Design review of the part built by this model. Coordinates are the model's own, in mm. A direction names the side the tool comes from. Give positions to 0.01 mm unless a question says otherwise; leave off trailing zeros. Loops run counter-clockwise (first coordinate to the right, second up) from the corner with the lowest first, then second, coordinate; pieces in that order, holes last. Notation, with made-up numbers: (-12, 63) -> (-1, 63) arc R18 ccw to (-1, 94) -> close; hole circle Ø9 at (78.5, 58). An arc over 180 degrees is marked (long way). Use a Markdown table: item, result. Add a question column.
1. For faces 1 (the flat face through (-256.279, 10.628, -40.025)), 2 (the cylindrical face through (-281.7, 4.2, -4)), list the 3-axis set-ups (+Z, -Z, +X, -X, +Y, -Y) from which the entire face can be reached by the end or side of a thin tool; tool diameter is ignored.
2. Add section A-A (x = -155). State the section outline as (y, z) points, and give its area (3 significant figures).
3. For pin 1 Ø0.9 at (x, y) = (-274.5, 24) entering from +Z; pin 2 Ø10 at (x, y) = (-470.5, 8) entering from +Z; pin 3 Ø12 at (x, z) = (-63, -6) entering from -Y, all flat-tipped, find the tip position at first contact; note any pin that passes through.
4. To check wall thickness, follow line 1 (Y direction, x = -477.5, z = -13); line 2 (Y direction, x = -232, z = -1.5); line 3 (X direction, y = 12.5, z = -14.5). State the ranges of each line that lie inside material, in increasing order.
```python
from build123d import *

# Parameters (mm, degrees)
F1_DEPTH      = 41
F1_DEPTH_BACK = 824
F5_DEPTH      = 824
F6_R          = 5
F8_DEPTH      = 52.001


with BuildPart() as f1:
    # F0 (on Right) → F1 (new body, two sides)
    with BuildSketch(Plane.YZ) as f1_sk:
        Polygon((22.4, 0), (0, 0), (0, -27), (20.4, -52), (25.4, -52), (25.4, -7), (22.4, -7), align=None)
    extrude(amount=F1_DEPTH)
    extrude(f1_sk.sketch, amount=-F1_DEPTH_BACK)

    # F2 (on Right) → F3 (revolve, cut)
    with BuildSketch(Plane.YZ):
        with BuildLine():
            ThreePointArc((0, -14), (4.100505, -4.100505), (14, 0))
            Line((14, 0), (14, 13.538237))
            Line((14, 13.538237), (0, 13.538237))
            Line((0, 13.538237), (0, -14))
        make_face()
    revolve(axis=Axis((0, 0, -0.230882), (0, 0, 1)), mode=Mode.SUBTRACT)

    # F4 (on face) → F5 (cut, through all)
    with BuildSketch(Plane(origin=(-824, 0, 0), x_dir=(0, -1, 0), z_dir=(-1, 0, 0))):
        with BuildLine():
            Line((-14, 13.538237), (-14, 0))
            ThreePointArc((-14, 0), (-4.100505, -4.100505), (0, -14))
            Line((0, -14), (0, 13.538237))
            Line((0, 13.538237), (-14, 13.538237))
        make_face()
    extrude(amount=-F5_DEPTH, mode=Mode.SUBTRACT)

    # F6
    f6_edges = [f1.edges().sort_by_distance(p)[0] for p in [
        (-391.5, 0, -27),
    ]]
    fillet(f6_edges, radius=F6_R)

    # F7 (on face) → F8 (cut, through all)
    with BuildSketch(Plane.XY):
        Polygon((-520.652341, -20.947659), (-567, 25.4), (-818.416774, 72.289795), (-858.546881, 112.419901), (-858.546881, -20.947659), align=None)
    extrude(amount=-F8_DEPTH, mode=Mode.SUBTRACT)


solid = f1.part
```
Taken from the geometry:
| question | item | result |
|---|---|---|
| 1 | face 1 | -Z, +X, -X, -Y |
| 1 | face 2 | +Z, -X, -Y |
| 2 | outline | (0, -25.22) arc R5 ccw to (1.13, -28.38) -> (20.4, -52) -> (25.4, -52) -> (25.4, -7) -> (22.4, -7) -> (22.4, 0) -> (14, 0) arc R14 ccw to (0, -14) -> close |
| 2 | area | 1,000 mm^2 |
| 3 | pin 1 | stops at z = -7 |
| 3 | pin 2 | stops at z = -0.04 |
| 3 | pin 3 | stops at y = 0.14 |
| 4 | line 1 | y = 0.04 to 25.4 |
| 4 | line 2 | y = 7.7 to 22.4 |
| 4 | line 3 | x = -554.1 to 41 |
